Design review of the part built by this model. Coordinates are the model's own, in mm. Coordinates: 2 decimals unless noted, no trailing zeros. Loops run counter-clockwise (first coordinate to the right, second up) from the corner with the lowest first, then second, coordinate; pieces in that order, holes last. Notation, with made-up numbers: (-6.5, 28.25) -> (41.5, 28.25) arc R18 ccw to (41.5, 57.25) -> close; hole circle Ø4 at (71.5, 13.25). An arc over 180 degrees is marked (long way). One line per item, written item: value. Start each with the question number.
1. Add section A-A on z = 3.25. Write out the cut boundary in (x, y), plus the area to 3 significant figures.
2. For probe 1 along X at (y, z) = (4.7, -3); probe 2 along Z at (x, y) = (25, 2.35); probe 3 along Y at (x, z) = (25.5, -0.75), list the stretches that pass through material, from the lowest coordinate up.
3. Add section B-B on x = -3. Write out the cut boundary in (y, z), plus the area to 3 significant figures.
4. Insertion check: pin 1 (1 mm diameter, centred on x = -11.5, z = -3, fed in from +Y). The pin has a flat end and moves straight along its axis. Give the tip position at first contact, or say it passes through.
5. Add section C-C on z = 0. Write out the cut boundary in (x, y), plus the area to 3 significant figures.
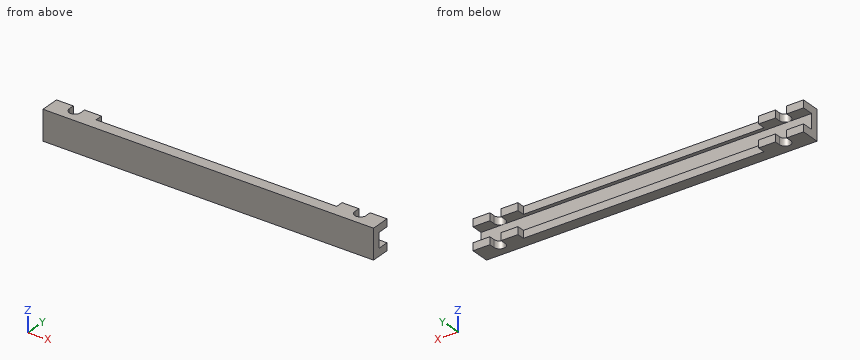
```python
from build123d import *

# Parameters (mm, degrees)
SKETCH1_W           = 44.1
SKETCH1_H           = 8
BOSS_EXTRUDE1_DEPTH = 2
SKETCH2_W           = 12
SKETCH2_H           = 2
BOSS_EXTRUDE2_DEPTH = 3
CUT_EXTRUDE1_DEPTH  = 46.097782651
SKETCH4_W           = 32.1
SKETCH4_H           = 2
BOSS_EXTRUDE3_DEPTH = 1


with BuildPart() as part:
    # Sketch1 → Boss-Extrude1 (new body)
    with BuildSketch(Plane(origin=(0, 0, 0), x_dir=(1, 0, 0), z_dir=(0, 1, 0))):
        with Locations((22.05, 0)):
            Rectangle(SKETCH1_W, SKETCH1_H)
    boss_extrude1 = extrude(amount=BOSS_EXTRUDE1_DEPTH)

    # Sketch2 → Boss-Extrude2 (add)
    with BuildSketch(Plane(origin=(0, 2, 0), x_dir=(1, 0, 0), z_dir=(0, 1, 0))):
        with Locations((38.1, 3)):
            Rectangle(SKETCH2_W, SKETCH2_H)
        with Locations((38.1, -3)):
            Rectangle(SKETCH2_W, SKETCH2_H)
    boss_extrude2 = extrude(amount=BOSS_EXTRUDE2_DEPTH)

    # Sketch3 → Cut-Extrude1 (cut, through all)
    with BuildSketch(Plane.XY.offset(4)):
        with BuildLine():
            Line((36.6, 3.5), (36.6, 5))
            Line((36.6, 5), (39.6, 5))
            Line((39.6, 5), (39.6, 3.5))
            ThreePointArc((39.6, 3.5), (38.1, 2), (36.6, 3.5))
        make_face()
    cut_extrude1 = extrude(amount=-CUT_EXTRUDE1_DEPTH, mode=Mode.SUBTRACT)

    # Sketch4 → Boss-Extrude3 (add)
    with BuildSketch(Plane(origin=(0, 2, 0), x_dir=(1, 0, 0), z_dir=(0, 1, 0))):
        with Locations((16.05, -3)):
            Rectangle(SKETCH4_W, SKETCH4_H)
        with Locations((16.05, 3)):
            Rectangle(SKETCH4_W, SKETCH4_H)
    boss_extrude3 = extrude(amount=BOSS_EXTRUDE3_DEPTH)

    # Mirror1: Boss-Extrude1, Boss-Extrude2, Cut-Extrude1, Boss-Extrude3 across plane
    add(boss_extrude1.mirror(Plane(origin=(0, 0, 0), x_dir=(0, 0, 1), z_dir=(1, 0, 0))))
    add(boss_extrude2.mirror(Plane(origin=(0, 0, 0), x_dir=(0, 0, 1), z_dir=(1, 0, 0))))
    add(cut_extrude1.mirror(Plane(origin=(0, 0, 0), x_dir=(0, 0, 1), z_dir=(1, 0, 0))), mode=Mode.SUBTRACT)
    add(boss_extrude3.mirror(Plane(origin=(0, 0, 0), x_dir=(0, 0, 1), z_dir=(1, 0, 0))))


solid = part.part
```
Worked answers:
1. outline: (-44.1, 0) -> (44.1, 0) -> (44.1, 5) -> (39.6, 5) -> (39.6, 3.5) arc R1.5 cw to (36.6, 3.5) -> (36.6, 5) -> (32.1, 5) -> (32.1, 3) -> (-32.1, 3) -> (-32.1, 5) -> (-36.6, 5) -> (-36.6, 3.5) arc R1.5 cw to (-39.6, 3.5) -> (-39.6, 5) -> (-44.1, 5) -> close
1. area: 297 mm²
2. probe 1: x = -44.1 to -39.6, -36.6 to -32.1, 32.1 to 36.6, 39.6 to 44.1
2. probe 2: z = -4 to -2, 2 to 4
2. probe 3: y = 0 to 2
3. outline: (0, -4) -> (3, -4) -> (3, -2) -> (2, -2) -> (2, 2) -> (3, 2) -> (3, 4) -> (0, 4) -> close
3. area: 20.0 mm²
4. pin 1: stops at y = 3
5. outline: (-44.1, 0) -> (44.1, 0) -> (44.1, 2) -> (-44.1, 2) -> close
5. area: 176 mm²
